Geometry check sheet. Reference: the model listing, model coordinates, mm. Face numbers are marked on the shaded views. A direction names the side the tool comes from. Give positions to 0.01 mm unless a question says otherwise; leave off trailing zeros. Write each loop counter-clockwise with the first axis right and the second up, starting at its lowest first coordinate (ties: lowest second). Pieces come first, ordered by that corner, then holes. Notation, with made-up numbers: (43.5, 14) -> (93.5, 14) arc R21 cw to (93.5, 22) -> close; hole circle Ø5 at (43.5, 33). An arc over 180 degrees is marked (long way). One line per item, written item: value.
from build123d import *

# Parameters (mm, degrees)
F1_DEPTH = 12
F2_DEPTH = 1


with BuildPart() as f1:
    # F0 (on Top) → F1 (new body)
    with BuildSketch(Plane.XY):
        Polygon((-6.8, -30.8), (6.8, -30.8), (6.8, 14.2), (16.8, 14.2), (16.8, 30.8), (6.8, 30.8), (-6.8, 30.8), align=None)
        Polygon((6, -30), (-6, -30), (-6, 30), (6, 30), (16, 30), (16, 15), (6, 15), align=None, mode=Mode.SUBTRACT)
    extrude(amount=F1_DEPTH)

    # F0 (on Top) → F2 (join)
    with BuildSketch(Plane.XY):
        Polygon((-6, 30), (-6, -30), (6, -30), (6, 15), (16, 15), (16, 30), (6, 30), align=None)
    extrude(amount=F2_DEPTH)


solid = f1.part
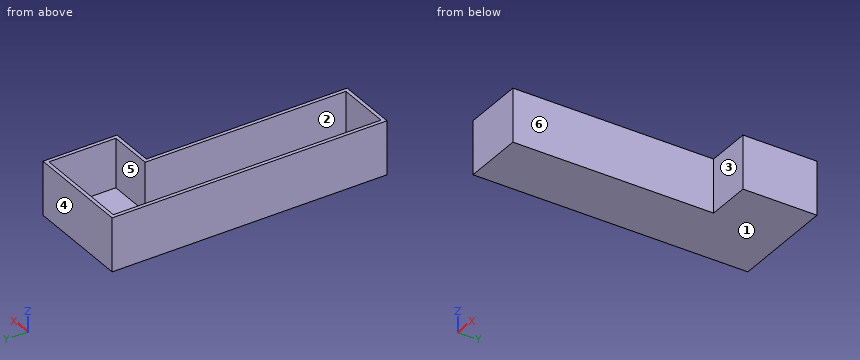
1) Scan lines: probe 1 along Y at (x, z) = (10.75, 3); probe 2 along Y at (x, z) = (3, 5); probe 3 along X at (y, z) = (21, 6.75). Record each from-to range of solid material in increasing order.
Verdict:
probe 1: 14.2 to 15, 30 to 30.8
probe 2: -30.8 to -30, 30 to 30.8
probe 3: -6.8 to -6, 16 to 16.8
2) Sectioned sample at A-A on z = 9.25. Record the cut outline in (x, y), plus the area to 3 significant figures.
Verdict:
outline: (-6.8, -30.8) -> (6.8, -30.8) -> (6.8, 14.2) -> (16.8, 14.2) -> (16.8, 30.8) -> (-6.8, 30.8) -> close; hole (-6, -30) -> (6, -30) -> (6, 15) -> (16, 15) -> (16, 30) -> (-6, 30) -> close
area: 134 mm^2
3) Mould release check, pull along X, two halves, no side actions. Record for the marked faces 4, 5 and 6: released by +X, released by -X, zero draft, split by the parting line, or undercut.
Verdict:
face 4: zero draft
face 5: undercut
face 6: released by +X
4) Sectioned sample at B-B on x = 5. Record the cut outline in (y, z), plus the area to 3 significant figures.
Verdict:
outline: (-30.8, 0) -> (30.8, 0) -> (30.8, 12) -> (30, 12) -> (30, 1) -> (-30, 1) -> (-30, 12) -> (-30.8, 12) -> close
area: 79.2 mm^2
5) Depth check by flat-ended pin: pin 1 Ø6 at (y, z) = (-11, 5.5) entering from +X; pin 2 Ø3 at (x, z) = (12.5, 8.5) entering from -Y; pin 3 Ø1 at (x, y) = (5, -1.5) entering from +Z. Enter the tip coordinate at first touch or a pass-through.
Verdict:
pin 1: x = 6.8
pin 2: y = 14.2
pin 3: z = 1
6) Sectioned sample at C-C on y = 22.5. Record the cut outline in (x, z).
Verdict:
outline: (-6.8, 0) -> (16.8, 0) -> (16.8, 12) -> (16, 12) -> (16, 1) -> (-6, 1) -> (-6, 12) -> (-6.8, 12) -> close
7) Tool access check on the marked faces 1, 2 and 3. Record the directions out of +Z, -Z, +X, -X, +Y, -Y that give a thin tool (end or side, any length) a straight path to the whole face; none if there is none.
Verdict:
face 1: -Z, +X, -X, +Y, -Y
face 2: +Z
face 3: +Z, -Z, +X, -Y
